Geometry: final body of the model. Coordinates: model frame, mm. Face numbers are marked on the shaded views. A direction names the side the tool comes from. Give positions to 0.01 mm unless a question says otherwise; leave off trailing zeros. Order: outer loops, then holes, each group sorted by start corner. A loop starts at its lowest first (then second) coordinate and runs counter-clockwise, first axis right, second up. Notation, with made-up numbers: (-23.75, -32) - (22.25, -32) arc R19 ccw to (22.25, -26) - close; hole circle Ø9 at (17.5, 57.25). An arc over 180 degrees is marked (long way). Use one line per item in the form item = value.
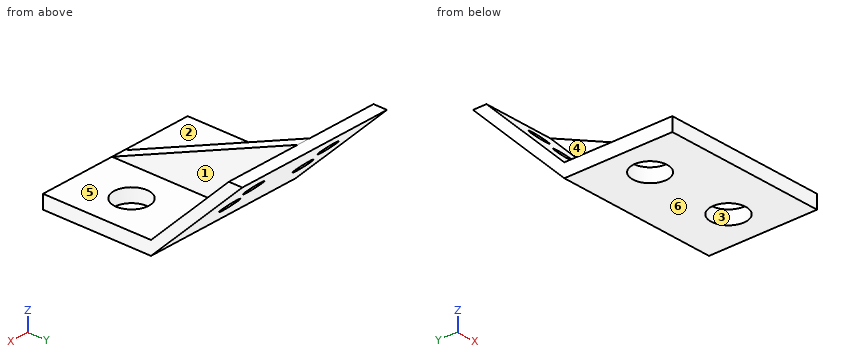
from build123d import *

# Parameters (mm, degrees)
F0_W      = 80
F0_H      = 10
F1_DEPTH  = 60
F2_W      = 10
F2_H      = 137.5997612298
F3_DEPTH  = 62.5
F5_DEPTH  = 25
F7_DEPTH  = 25
F8_R      = 7
F9_DEPTH  = 54.8723173841
F10_R     = 12.8351278785
F11_DEPTH = 10.001
F12_R     = 12.7228131032
F13_DEPTH = 10.001


with BuildPart() as f1:
    # F0 (on Right) → F1 (new body, symmetric)
    with BuildSketch(Plane.YZ):
        Rectangle(F0_W, F0_H)
        Polygon((40, 5), (40, -5), (107.5997612298, 62.5997612298), (97.5997612298, 62.5997612298), align=None)
    extrude(amount=F1_DEPTH, both=True)

    # F2 (on Top) → F3 (join)
    with BuildSketch(Plane.XY):
        with Locations((-2.2415908799, 28.7998806149)):
            Rectangle(F2_W, F2_H)
    extrude(amount=F3_DEPTH)

    # F4 (on face) → F5 (cut)
    with BuildSketch(Plane.YZ.offset(2.7584091201)):
        Polygon((-40, 62.5), (-40, 5), (97.5, 62.5), align=None)
    extrude(amount=-F5_DEPTH, mode=Mode.SUBTRACT)

    # F6 (on face) → F7 (cut)
    with BuildSketch(Plane.YZ.offset(2.7584091201)):
        Polygon((97.5997612298, 52.5997612298), (45, 0), (97.5997612298, 0), align=None)
    extrude(amount=-F7_DEPTH, mode=Mode.SUBTRACT)

    # F8 (on face) → F9 (cut, through all)
    with BuildSketch(Plane(origin=(0, 17.5, -17.5), x_dir=(1, 0, 0), z_dir=(0, -0.7071067812, 0.7071067812))):
        with Locations((26.0520085543, 89.2042198464)):
            Circle(F8_R)
        with Locations((27.1440549599, 65.627058422)):
            Circle(F8_R)
        with Locations((-35.6482013747, 89.2042198464)):
            Circle(F8_R)
        with Locations((-33.7371340773, 65.627058422)):
            Circle(F8_R)
    extrude(amount=-F9_DEPTH, mode=Mode.SUBTRACT)

    # F10 (on face) → F11 (cut, through all)
    with BuildSketch(Plane.XY.offset(5)):
        with Locations((31.3792045601, 0)):
            Circle(F10_R)
    extrude(amount=-F11_DEPTH, mode=Mode.SUBTRACT)

    # F12 (on face) → F13 (cut, through all)
    with BuildSketch(Plane.XY.offset(5)):
        with Locations((-33.6207954399, 0)):
            Circle(F12_R)
    extrude(amount=-F13_DEPTH, mode=Mode.SUBTRACT)


solid = f1.part
(1) Cut plane A-A on z = 2.5. Output: boundary loops of the cut face in (x, y), plus the area to 3 significant figures.
Computed values:
outline = (-60, -40) - (60, -40) - (60, 47.5) - (-60, 47.5) - close; hole circle Ø25.45 at (-33.62, 0); hole circle Ø25.67 at (31.38, 0)
area = 9,470 mm²
(2) Reachability of the marked faces 4, 5 and 6 from +Z, -Z, +X, -X, +Y, -Y: full face, straight path, thin tool, end or side. Return the list, or none.
Computed values:
face_4 = +Z, -X, -Y
face_5 = +Z, +X, -Y
face_6 = -Z, +X, -X, +Y, -Y
(3) Cut plane C-C on x = 12.5. Output: boundary loops of the cut face in (y, z).
Computed values:
outline = (-40, -5) - (40, -5) - (107.6, 62.6) - (97.6, 62.6) - (40, 5) - (-40, 5) - close
(4) Cut plane D-D on y = 22. Output: boundary loops of the cut face in (x, z), plus the area to 3 significant figures.
Computed values:
outline = (-60, -5) - (60, -5) - (60, 5) - (2.76, 5) - (2.76, 30.93) - (-7.24, 30.93) - (-7.24, 5) - (-60, 5) - close
area = 1,460 mm²
(5) Cut plane B-B on y = 0. Output: boundary loops of the cut face in (x, z).
Computed values:
outline = (-60, -5) - (-46.34, -5) - (-46.34, 5) - (-60, 5) - close; (-20.9, -5) - (18.54, -5) - (18.54, 5) - (2.76, 5) - (2.76, 21.73) - (-7.24, 21.73) - (-7.24, 5) - (-20.9, 5) - close; (44.21, -5) - (60, -5) - (60, 5) - (44.21, 5) - close
(6) Ray query, line 1 along X through (y, z) = (8.5, 9); line 2 along Z through (x, y) = (44, -17.5); line 3 along Z through (x, y) = (-42, 60.5). Return the intervals inside material, ascending.
Computed values:
line_1 = -7.24 to 2.76
line_2 = -5 to 5
line_3 = 15.5 to 25.5
(7) Pull-direction query (X, two-part tool) for the marked faces 1, 2 and 3; classes: released by +X, released by -X, zero draft, split by the parting line, or undercut.
Computed values:
face_1 = released by +X
face_2 = zero draft
face_3 = undercut
(8) Contact query for flat-ended pins moving along their axis: pin 1 Ø2 at (x, z) = (38, 26.5) entering from +Y; pin 2 Ø5 at (x, y) = (-45.5, 71.5) entering from +Z; pin 3 Ø12 at (x, y) = (-30, 55) entering from -Z. Output: stop coordinate, or through.
Computed values:
pin_1 = 72.5
pin_2 = 39
pin_3 = 4
